from build123d import *

# Parameters (mm, degrees)
SKETCH2_W                    = 140
SKETCH2_H                    = 230
BASE_FLANGE1_DEPTH           = 2
EDGE_FLANGE1_STRIP_W         = 9.4732
EDGE_FLANGE1_STRIP_H         = 2
EDGE_FLANGE1_STRIP_CUT_DEPTH = 230
EDGE_FLANGE1_DEPTH           = 230
F_5_0_5_DIAMETER_HOLE1_D     = 5
F_5_0_5_DIAMETER_HOLE1_DEPTH = 144


# Sheet-metal steps are written as plain solids
with BuildPart() as part:
    # Sketch2 → Base-Flange1 (new body)
    with BuildSketch(Plane(origin=(0, 0, 0), x_dir=(1, 0, 0), z_dir=(0, 1, 0))):
        Rectangle(SKETCH2_W, SKETCH2_H)
    extrude(amount=BASE_FLANGE1_DEPTH)

    # Edge-Flange1 strip (across the edge) → Edge-Flange1 strip cut (cut)
    with BuildSketch(Plane(origin=(70, 0, -115), x_dir=(-1, 0, 0), z_dir=(0, 0, 1))):
        with Locations((-4, -1)):
            Rectangle(EDGE_FLANGE1_STRIP_W, EDGE_FLANGE1_STRIP_H)
    edge_flange1_strip_cut = extrude(amount=EDGE_FLANGE1_STRIP_CUT_DEPTH, mode=Mode.SUBTRACT)

    # Edge-Flange1 section (across the edge) → Edge-Flange1 (add)
    with BuildSketch(Plane(origin=(70, 0, -115), x_dir=(-1, 0, 0), z_dir=(0, 0, 1))):
        with BuildLine():
            Line((-2, 0.7366), (-2, 101))
            Line((-2, 101), (0, 101))
            Line((0, 101), (0, 0.7366))
            ThreePointArc((0, 0.7366), (0.215745145, 0.215745145), (0.7366, 0))
            Line((0.7366, 0), (0.7366, -2))
            ThreePointArc((0.7366, -2), (-1.198468417, -1.198468417), (-2, 0.7366))
        make_face()
    edge_flange1 = extrude(amount=EDGE_FLANGE1_DEPTH)

    # Ø5.0 (5) Diameter Hole1
    with Locations(Plane(origin=(72, 0, 0), x_dir=(0, 0, -1), z_dir=(1, 0, 0))):
        with Locations((0, -91), (80, -91), (-80, -91)):
            f_5_0_5_diameter_hole1 = Hole(F_5_0_5_DIAMETER_HOLE1_D / 2, depth=F_5_0_5_DIAMETER_HOLE1_DEPTH)

    # Mirror1: Edge-Flange1 strip cut, Edge-Flange1, Ø5.0 (5) Diameter Hole1 across plane
    add(edge_flange1_strip_cut.mirror(Plane(origin=(0, 0, 0), x_dir=(0, 0, 1), z_dir=(1, 0, 0))), mode=Mode.SUBTRACT)
    add(edge_flange1.mirror(Plane(origin=(0, 0, 0), x_dir=(0, 0, 1), z_dir=(1, 0, 0))))
    add(f_5_0_5_diameter_hole1.mirror(Plane(origin=(0, 0, 0), x_dir=(0, 0, 1), z_dir=(1, 0, 0))), mode=Mode.SUBTRACT)


solid = part.part
CAD build for the part. Positions are in the model's coordinates, mm. A direction names the side the tool comes from. Round coordinates to 2 decimals unless told otherwise and drop trailing zeros. Write each loop counter-clockwise with the first axis right and the second up, starting at its lowest first coordinate (ties: lowest second). Pieces come first, ordered by that corner, then holes. Notation, with made-up numbers: M 85,59.5 L 133,59.5 A23 cw 133,82.5 Z; hole C 43,59 d6. An arc over 180 degrees is marked long. Put each result on its own line as item: value. Start each with the question number.
1) Pin check, flat tip, straight feed: pin 1 Ø3 at (y, z) = (-91, 0) entering from +X. Stop position of the tip, or through.
2) Saw through at A-A, the plane y = -15. Write the cut outline in (x, z).
3) 3-axis set-ups, long thin cutter, end or side, ignore diameter. For faces 1 (the flat face through (-70, -52, -2)), 2 (the cylindrical face through (-70.99, -88.52, -80.33)): which of +Z, -Z, +X, -X, +Y, -Y reach the whole face in a straight line?
4) Pull direction Y, two halves, no side cores. Call faces 3 (the flat face through (70, -52, -2)), 4 (the cylindrical face through (70.99, -88.52, 79.67)), 5 (the cylindrical face through (70.99, -88.52, -0.33)), 6 (the flat face through (-1, 0, -2)): pulls with the +Y half, pulls with the -Y half, needs draft (parallel to the pull), parting line crosses it, or undercut.
5) Saw through at C-C, the plane y = -91. Count the separate pieces of the cut face and the enclosed holes in it, and give its area (3 significant figures).
6) Saw through at D-D, the plane z = 53.5. Write the cut outline in (x, y), and give its area (3 significant figures).
7) Saw through at B-B, the plane z = 80. Write the cut outline in (x, y).
8) Drill centre lines: probe 1 along Z at (x, y) = (-70.55, -91); probe 2 along X at (y, z) = (-47, 101); probe 3 along Y at (x, z) = (-35, 101). Where is each one in solid material? Low to high. Write a range as [from, to].
Resolved:
1. pin 1: through
2. outline: M -72,-115 L -70,-115 L -70,115 L -72,115 Z; M 70,-115 L 72,-115 L 72,115 L 70,115 Z
3. face 1: +Z, -Z, -Y
3. face 2: +X, -X
4. face 3: needs draft
4. face 4: undercut
4. face 5: undercut
4. face 6: pulls with the -Y half
5. separate pieces: 8
5. enclosed holes: 0
5. area: 860 mm²
6. outline: M -72,-101 L -70,-101 L -70,-0.74 A0.74 cw -69.26,0 L 69.26,0 A0.74 cw 70,-0.74 L 70,-101 L 72,-101 L 72,-0.74 A2.74 ccw 69.26,2 L -69.26,2 A2.74 ccw -72,-0.74 Z
6. area: 689 mm²
7. outline: M -72,-101 L -70,-101 L -70,-93.5 L -72,-93.5 Z; M -72,-88.5 L -70,-88.5 L -70,-0.74 A0.74 cw -69.26,0 L 69.26,0 A0.74 cw 70,-0.74 L 70,-88.5 L 72,-88.5 L 72,-0.74 A2.74 ccw 69.26,2 L -69.26,2 A2.74 ccw -72,-0.74 Z; M 70,-101 L 72,-101 L 72,-93.5 L 70,-93.5 Z
8. probe 1: [-115, -82.5], [-77.5, -2.5], [2.5, 77.5], [82.5, 115]
8. probe 2: [-72, -70], [70, 72]
8. probe 3: [0, 2]
